```python
from build123d import *

# Parameters (mm, degrees)
EXTRUDE_1_DEPTH     = 4
SKETCH_2_R          = 2.5
EXTRUDE_2_DEPTH     = 16
SKETCH_3_OUTSIDE_W  = 70.114
SKETCH_3_OUTSIDE_H  = 71.352
SKETCH_3_OUTSIDE_R  = 4
CUT_EXTRUDE_1_DEPTH = 16
CUT_EXTRUDE_1_DRAFT = -60


# Read off the part's stored shape, not the designer's step: #10-24 机械螺纹 螺柱4
with BuildPart() as part:
    # 草图1 → 凸台-拉伸1 (new body)
    with BuildSketch(Plane(origin=(0, 0, 0), x_dir=(1, 0, 0), z_dir=(0, 1, 0))):
        Polygon((4, -2.309401077), (4, 2.309401077), (0, 4.618802154), (-4, 2.309401077), (-4, -2.309401077), (0, -4.618802154), align=None)
    extrude(amount=EXTRUDE_1_DEPTH)

    # 草图2 → 凸台-拉伸2 (add)
    with BuildSketch(Plane.XZ):
        with Locations(Location((0, 0, 0), (0, 0, 270))):
            Circle(SKETCH_2_R)
    extrude(amount=EXTRUDE_2_DEPTH)


with BuildPart() as cut_extrude_1_tool:
    # 草图3 outside → 切除-拉伸1 (with draft: the straight prism first)
    with BuildSketch(Plane(origin=(0, 4, 0), x_dir=(1, 0, 0), z_dir=(0, 1, 0))):
        Rectangle(SKETCH_3_OUTSIDE_W, SKETCH_3_OUTSIDE_H)
        Circle(SKETCH_3_OUTSIDE_R, mode=Mode.SUBTRACT)
    extrude(amount=-CUT_EXTRUDE_1_DEPTH)
    # 切除-拉伸1: the draft: its side faces are tilted about the plane it starts from
    cut_extrude_1_sides = [cut_extrude_1_tool.faces().sort_by_distance(p)[0] for p in [
        (0, -4, 35.676),
        (35.057, -4, 0),
        (0, -4, -35.676),
        (-35.057, -4, 0),
        (-4, -4, 0),
    ]]
    draft(cut_extrude_1_sides, Plane(origin=(0, 4, 0), x_dir=(1, 0, 0), z_dir=(0, 1, 0)), CUT_EXTRUDE_1_DRAFT)


with BuildPart() as part_1:
    add(part.part)

    # 切除-拉伸1: cut by cut_extrude_1_tool
    add(cut_extrude_1_tool.part, mode=Mode.SUBTRACT)

    # #10-24 机械螺纹 螺柱4 outline → #10-24 机械螺纹 螺柱4 (revolve, cut)
    with BuildSketch(Plane.XY):
        Polygon((1.78308, -16), (2.5, -16), (2.5, -6), (2.413, -6), (2.413, -15.37008), align=None)
    revolve(axis=Axis((0, 0, 0), (0, 1, 0)), mode=Mode.SUBTRACT)


solid = part_1.part
```
For this review, take the finished solid that the model builds, in its own axes (mm). A direction names the side the tool comes from. Round coordinates to 2 decimals unless told otherwise and drop trailing zeros. Write each loop counter-clockwise with the first axis right and the second up, starting at its lowest first coordinate (ties: lowest second). Pieces come first, ordered by that corner, then holes.
1) Take a section at B-B on y = -9. Give the boundary of the cut face in (x, z).
Answer below:
outline: circle Ø4.83 at (0, 0)
2) Take a section at C-C on y = -5.5. Give the boundary of the cut face in (x, z), then the cut area to 3 significant figures.
Answer below:
outline: circle Ø5 at (0, 0)
area: 19.6 mm2
3) Insertion check: pin 1 Ø5 at (y, z) = (-3.5, -2.5) entering from +X; pin 2 Ø3 at (y, z) = (-3.5, 2.5) entering from -X; pin 3 Ø4 at (x, y) = (-1, -9) entering from -Z. Each pin has a flat end and moves straight along its axis. Give the tip position at first contact, or say it passes through.
Answer below:
pin 1: stops at x = 2.5
pin 2: stops at x = -2.29
pin 3: stops at z = -2.41
4) For line 1 along Y through (x, z) = (-0.75, 2.75); line 2 along Z through (x, y) = (0, -14.5), list the stretches that pass through material, from the lowest coordinate up.
Answer below:
line 1: y = 0 to 4
line 2: z = -2.41 to 2.41
5) Machinability: for faces 1 (the face through (-2.44, -2.96, 0.54)), 2 (the face through (-3.597, 3.915, 2.065)), which of the approach directions +Z, -Z, +X, -X, +Y, -Y give a long, thin tool a straight path to every point of the face, cutting with its end or side? Answer none if there is none.
Answer below:
face 1: -Y
face 2: +Z, -X, +Y
6) Take a section at A-A on y = 1.5. Give the boundary of the cut face in (x, z), then the cut area to 3 significant figures.
Answer below:
outline: (-4, -2.31) - (0, -4.62) - (4, -2.31) - (4, 2.31) - (0, 4.62) - (-4, 2.31) - close
area: 55.4 mm2
